from build123d import *

# Parameters (mm, degrees)
F1_DEPTH  = 2.15
F2_W      = 12.4
F2_H      = 19.3
F3_DEPTH  = 2.15
F4_DEPTH  = 2.15
F6_DEPTH  = 25
F7_DEPTH  = 2.15
F9_DEPTH  = 25
F11_DEPTH = 12.4
F13_DEPTH = 2.5
F14_DEPTH = 1.3
F16_DEPTH = 2.5


with BuildPart() as f1:
    # F0 (on Top) → F1 (new body)
    with BuildSketch(Plane.XY):
        Polygon((12.4, 0), (0, 0), (0, -6), (0, -9), (6.2, -9), (12.4, -9), (12.4, -6), align=None)
        Polygon((0, -9), (0, -6), (-0.4, -9), align=None)
        Polygon((12.8, -9), (12.4, -6), (12.4, -9), align=None)
        Polygon((6.2, -9), (0, -9), (0, -13), (0, -16), (6.2, -16), (12.4, -16), (12.4, -13), (12.4, -9), align=None)
        Polygon((0, -16), (0, -13), (-0.4, -16), align=None)
        Polygon((12.8, -16), (12.4, -13), (12.4, -16), align=None)
        Polygon((6.2, -16), (0, -16), (0, -18), (12.4, -18), (12.4, -16), align=None)
    extrude(amount=F1_DEPTH)

    # F2 (on face) → F3 (join)
    with BuildSketch(Plane.XY.offset(2.15)):
        with Locations((6.2, -9.65)):
            Rectangle(F2_W, F2_H)
    extrude(amount=F3_DEPTH)

    # F4 (add): a face of the model
    f4_faces = [f1.faces().sort_by_distance(p)[0] for p in [
        (12.5333333333, -8, 2.15),
    ]]
    extrude(f4_faces, amount=F4_DEPTH)

    # F5 (on face) → F6 (cut)
    with BuildSketch(Plane.YZ.offset(12.4)):
        Polygon((-9, 4.3), (-9, 2.15), (-7.8, 4.3), align=None)
    extrude(amount=F6_DEPTH, mode=Mode.SUBTRACT)

    # F7 (add): a face of the model
    f7_faces = [f1.faces().sort_by_distance(p)[0] for p in [
        (-0.1333333333, -15, 2.15),
    ]]
    extrude(f7_faces, amount=F7_DEPTH)

    # F8 (on face) → F9 (cut)
    with BuildSketch(Plane(origin=(0, 0, 0), x_dir=(0, -1, 0), z_dir=(-1, 0, 0))):
        Polygon((14.8, 4.3), (16, 2.15), (16, 4.3), align=None)
    extrude(amount=F9_DEPTH, mode=Mode.SUBTRACT)

    # F10 (on face) → F11 (join, through all)
    with BuildSketch(Plane.YZ.offset(12.4)):
        Polygon((1.1, 4.3), (0, 4.3), (0, 2.15), align=None)
    extrude(amount=-F11_DEPTH)

    # F12 (on face) → F13 (join)
    with BuildSketch(Plane.XZ.offset(19.3)):
        with BuildLine():
            Line((0, 2.15), (2.15, 2.15))
            ThreePointArc((2.15, 2.15), (0, 4.3), (-2.15, 2.15))
            Line((-2.15, 2.15), (0, 2.15))
        make_face()
        with BuildLine():
            Line((10.25, 2.15), (2.15, 2.15))
            ThreePointArc((2.15, 2.15), (1.5202795796, 0.6297204204), (0, 0))
            Line((0, 0), (12.4, 0))
            ThreePointArc((12.4, 0), (10.8797204204, 0.6297204204), (10.25, 2.15))
        make_face()
        with BuildLine():
            ThreePointArc((0, 0), (1.5202795796, 0.6297204204), (2.15, 2.15))
            Line((2.15, 2.15), (0, 2.15))
            Line((0, 2.15), (-2.15, 2.15))
            ThreePointArc((-2.15, 2.15), (-1.5202795796, 0.6297204204), (0, 0))
        make_face()
        with BuildLine():
            Line((12.4, 2.15), (10.25, 2.15))
            ThreePointArc((10.25, 2.15), (10.8797204204, 0.6297204204), (12.4, 0))
            ThreePointArc((12.4, 0), (13.9202795796, 0.6297204204), (14.55, 2.15))
            Line((14.55, 2.15), (12.4, 2.15))
        make_face()
        with BuildLine():
            ThreePointArc((14.55, 2.15), (12.4, 4.3), (10.25, 2.15))
            Line((10.25, 2.15), (12.4, 2.15))
            Line((12.4, 2.15), (14.55, 2.15))
        make_face()
        with BuildLine():
            ThreePointArc((0, 4.3), (1.5202795796, 3.6702795796), (2.15, 2.15))
            Line((2.15, 2.15), (10.25, 2.15))
            ThreePointArc((10.25, 2.15), (10.8797204204, 3.6702795796), (12.4, 4.3))
            Line((12.4, 4.3), (0, 4.3))
        make_face()
    extrude(amount=F13_DEPTH)

    # F12 (on face) → F14 (join)
    with BuildSketch(Plane.XZ.offset(19.3)):
        with BuildLine():
            ThreePointArc((0, 0), (1.5202795796, 0.6297204204), (2.15, 2.15))
            Line((2.15, 2.15), (0, 2.15))
            Line((0, 2.15), (-2.15, 2.15))
            ThreePointArc((-2.15, 2.15), (-1.5202795796, 0.6297204204), (0, 0))
        make_face()
        with BuildLine():
            Line((10.25, 2.15), (2.15, 2.15))
            ThreePointArc((2.15, 2.15), (1.5202795796, 0.6297204204), (0, 0))
            Line((0, 0), (12.4, 0))
            ThreePointArc((12.4, 0), (10.8797204204, 0.6297204204), (10.25, 2.15))
        make_face()
        with BuildLine():
            Line((12.4, 2.15), (10.25, 2.15))
            ThreePointArc((10.25, 2.15), (10.8797204204, 0.6297204204), (12.4, 0))
            ThreePointArc((12.4, 0), (13.9202795796, 0.6297204204), (14.55, 2.15))
            Line((14.55, 2.15), (12.4, 2.15))
        make_face()
    extrude(amount=-F14_DEPTH)

    # F15 (on face) → F16 (join)
    with BuildSketch(Plane.XZ.offset(21.8)):
        with BuildLine():
            ThreePointArc((12.4, -0.2), (14.75, 2.15), (12.4, 4.5))
            Line((12.4, 4.5), (0, 4.5))
            ThreePointArc((0, 4.5), (-2.35, 2.15), (0, -0.2))
            Line((0, -0.2), (12.4, -0.2))
        make_face()
    extrude(amount=-F16_DEPTH)


solid = f1.part
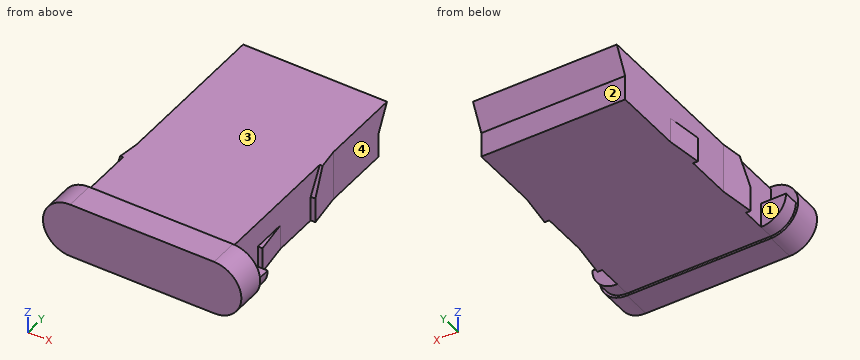
Build history of the part. All positions in model axes, mm. Face numbers are marked on the shaded views. A direction names the side the tool comes from. Round coordinates to 2 decimals unless told otherwise and drop trailing zeros. Write each loop counter-clockwise with the first axis right and the second up, starting at its lowest first coordinate (ties: lowest second). Pieces come first, ordered by that corner, then holes. Notation, with made-up numbers: (-9.5, 23) - (-2.5, 23) arc R24 ccw to (-2.5, 40) - close; hole circle Ø4 at (39.25, -10). An arc over 180 degrees is marked (long way). Use CSV: the item, a comma, the result in double quotes.
(1) Band-saw the part on D-D (z = 3.2). Write the cut outline in (x, y), plus the area to 3 significant figures.
Response:
outline,"(-2.1, -21.8) - (14.5, -21.8) - (14.5, -19.3) - (12.4, -19.3) - (12.4, -8.41) - (12.72, -8.41) - (12.4, -6) - (12.4, 0.54) - (0, 0.54) - (0, -13) - (-0.32, -15.41) - (0, -15.41) - (0, -19.3) - (-2.1, -19.3) - close"
area,"288 mm²"
(2) Band-saw the part on B-B (z = 1.8). Write the cut outline in (x, y).
Response:
outline,"(-2.32, -21.8) - (14.72, -21.8) - (14.72, -19.3) - (14.52, -19.3) - (14.52, -18) - (12.4, -18) - (12.4, -16) - (12.8, -16) - (12.4, -13) - (12.4, -9) - (12.8, -9) - (12.4, -6) - (12.4, 0) - (0, 0) - (0, -6) - (-0.4, -9) - (0, -9) - (0, -13) - (-0.4, -16) - (0, -16) - (0, -18) - (-2.12, -18) - (-2.12, -19.3) - (-2.32, -19.3) - close"
(3) Band-saw the part on A-A (x = 4.5). Write the cut outline in (y, z).
Response:
outline,"(-21.8, -0.2) - (-19.3, -0.2) - (-19.3, 0) - (0, 0) - (0, 2.15) - (1.1, 4.3) - (-19.3, 4.3) - (-19.3, 4.5) - (-21.8, 4.5) - close"
(4) Pin check, flat tips, straight feed: P1, Ø0.7, axis at x = 13, y = -18.5, coming from the +Z side; P2, Ø0.6, axis at x = 8.5, z = 1, coming from the +Y side; P3, Ø10, axis at x = 1.5, y = -1, coming from the +Z side. Stop position of each tip, or through.
Response:
P1,"z = 2.15"
P2,"y = 0"
P3,"z = 4.3"
(5) Wall check: line 1 (Y direction, x = 7.75, z = 0.85); line 2 (Z direction, x = 9.5, y = -4.75); line 3 (Y direction, x = -0.5, z = 3.35). Give the ranges that are in metal, low to high.
Response:
line 1,"-21.8 to 0"
line 2,"0 to 4.3"
line 3,"-21.8 to -19.3"
(6) Band-saw the part on C-C (y = -10.75). Write the cut outline in (x, z).
Response:
outline,"(0, 0) - (12.4, 0) - (12.4, 4.3) - (0, 4.3) - close"
(7) 3-axis set-ups, long thin cutter, end or side, ignore diameter. For the marked faces 1, 2, 3 and 4: which of +Z, -Z, +X, -X, +Y, -Y reach the whole face in a straight line?
Response:
face 1,"+Z, -Z, -X"
face 2,"-Z, +X, -X, +Y"
face 3,"+Z, +X, -X, +Y"
face 4,"+Z, -Z, +X, +Y"
